from build123d import *

# Parameters (mm, degrees)
SKETCH_1_R           = 7
EXTRUDE_1_DEPTH      = 34
EXTRUDE_2_DEPTH      = 2
EXTRUDE_2_DEPTH_BACK = 3
SKETCH_2_R           = 12
SKETCH_3_W           = 50
SKETCH_3_H           = 50
EXTRUDE_4_DEPTH      = 3
SKETCH_5_R           = 1.05
SKETCH_5_R_2         = 1
CUT_EXTRUDE_1_DEPTH  = 5
FILLET_1_R           = 10


with BuildPart() as part:
    # 草图1 → 凸台-拉伸1 (new body)
    with BuildSketch(Plane.XY):
        with Locations((-86.606649797, -63.783530386)):
            Circle(SKETCH_1_R)
    extrude(amount=EXTRUDE_1_DEPTH)

    # 草图2 → 凸台-拉伸2 (add, two sides: drawn at the far end of the back side and taken through both)
    with BuildSketch(Plane.XY.offset(34).offset(-EXTRUDE_2_DEPTH_BACK)):
        with Locations((-86.606649797, -63.783530386)):
            Circle(SKETCH_2_R)
    extrude(amount=EXTRUDE_2_DEPTH + EXTRUDE_2_DEPTH_BACK)

    # 草图3 → 凸台-拉伸4 (add)
    with BuildSketch(Plane.XY.offset(36)):
        with Locations((-79.849508923, -74.381256309)):
            Rectangle(SKETCH_3_W, SKETCH_3_H)
    extrude(amount=EXTRUDE_4_DEPTH)

    # 草图5 → 切除-拉伸1 (cut)
    with BuildSketch(Plane.XY.offset(39)):
        with Locations((-84.106649797, -86.087855448)):
            Circle(SKETCH_5_R)
        with Locations((-74.106649797, -86.087855448)):
            Circle(SKETCH_5_R_2)
        with Locations((-64.106649797, -86.087855448)):
            Circle(SKETCH_5_R_2)
        with Locations((-64.106649797, -76.087855448)):
            Circle(SKETCH_5_R_2)
        with Locations((-64.106649797, -66.087855448)):
            Circle(SKETCH_5_R)
        with Locations((-84.106649797, -66.087855448)):
            Circle(SKETCH_5_R)
    extrude(amount=-CUT_EXTRUDE_1_DEPTH, mode=Mode.SUBTRACT)

    # 圆角1
    fillet_1_edges = [part.edges().sort_by_distance(p)[0] for p in [
        (-104.849508923, -49.381256309, 37.5),
        (-104.849508923, -99.381256309, 37.5),
        (-54.849508923, -99.381256309, 37.5),
        (-54.849508923, -49.381256309, 37.5),
    ]]
    fillet(fillet_1_edges, radius=FILLET_1_R)


solid = part.part
Geometry: final body of the model. Coordinates: model frame, mm. A direction names the side the tool comes from. Give positions to 0.01 mm unless a question says otherwise; leave off trailing zeros. Write each loop counter-clockwise with the first axis right and the second up, starting at its lowest first coordinate (ties: lowest second). Pieces come first, ordered by that corner, then holes. Notation, with made-up numbers: (32.25, -34.75) -> (39.25, -34.75) arc R24 cw to (39.25, -17.75) -> close; hole circle Ø2 at (48, -21). An arc over 180 degrees is marked (long way). Answer as a JSON object with one key per item and string values.
1. Access query for faces 1 (the cylindrical face through (-102, -52.39, 37.52)), 2 (the flat face through (-81, -69, 31)). Directions: +Z, -Z, +X, -X, +Y, -Y. A direction counts if a zero-diameter tool reaches every point of the face in a straight line with its end or side. Return the directions, or none.
Ans:
{"face 1": "+Z, -Z, -X, +Y", "face 2": "-Z"}
2. Contact query for flat-ended pins moving along their axis: pin 1 (10 mm diameter, centred on x = -93.5, z = 13.5, fed in from +Y); pin 2 (6 mm diameter, centred on y = -72.5, z = 9.5, fed in from +X); pin 3 (12 mm diameter, centred on x = -80, z = 15.5, fed in from +Y). Output: stop coordinate, or through.
Ans:
{"pin 1": "stops at y = -57.04", "pin 2": "stops at x = -82.57", "pin 3": "stops at y = -56.81"}
3. Ray query, probe 1 along Z at (x, y) = (-62, -81); probe 2 along Z at (x, y) = (-93, -58); probe 3 along X at (y, z) = (-69, 14). Return the intervals inside material, ascending. Write a range as from..to.
Ans:
{"probe 1": "z = 36..39", "probe 2": "z = 31..39", "probe 3": "x = -91.27..-81.94"}
4. Cut plane B-B on y = -83. Output: boundary loops of the cut face in (x, z), and give its area (3 significant figures).
Ans:
{"outline": "(-104.85, 36) -> (-54.85, 36) -> (-54.85, 39) -> (-104.85, 39) -> close", "area": "150 mm^2"}
5. Cut plane A-A on x = -77.5. Output: boundary loops of the cut face in (y, z).
Ans:
{"outline": "(-99.38, 36) -> (-71.6, 36) -> (-71.6, 31) -> (-55.97, 31) -> (-55.97, 36) -> (-49.38, 36) -> (-49.38, 39) -> (-99.38, 39) -> close"}
6. Cut plane D-D on z = 30. Output: boundary loops of the cut face in (x, y), and give its area (3 significant figures).
Ans:
{"outline": "circle Ø14 at (-86.61, -63.78)", "area": "154 mm^2"}
7. Mould query, pull axis Y, two halves, no side actions, for faces 3 (the flat face through (-104.85, -75, 37)), 4 (the cylindrical face through (-57.857, -96.53, 37.521)), 5 (the flat face through (-84, -66, 34)). Classes: pulls with the +Y half, pulls with the -Y half, needs draft (parallel to the pull), parting line crosses it, or undercut.
Ans:
{"face 3": "needs draft", "face 4": "pulls with the -Y half", "face 5": "undercut"}
8. Cut plane C-C on z = 35. Output: boundary loops of the cut face in (x, y), and give its area (3 significant figures).
Ans:
{"outline": "circle Ø24 at (-86.61, -63.78); hole circle Ø2.1 at (-84.11, -66.09)", "area": "449 mm^2"}
